Design review of the part shown in the three views and the two pictorial views. Dimensions are in mm from the part's minimum x, y and z. Coordinates: 2 decimals unless noted, no trailing zeros. Order: outer loops, then holes, each group sorted by start corner. A loop starts at its lowest first (then second) coordinate and runs counter-clockwise, first axis right, second up. Notation, with made-up numbers: (11.5, -2.75) -> (60.5, -2.75) arc R34 cw to (60.5, 29.25) -> close; hole circle Ø5 at (68.25, 42). An arc over 180 degrees is marked (long way). Write item = value, one per line. Start each with the question number.
1) Consider section C-C on z = 7. Give the boundary of the cut face in (x, y), and give its area (3 significant figures).
2) Insertion check: pin 1 Ø2 at (y, z) = (63, 6) entering from -X; pin 2 Ø2 at (x, z) = (31.5, 7) entering from -Y; pin 3 Ø4 at (x, z) = (16.5, 4.5) entering from +Y. Each pin has a flat end and moves straight along its axis. Give the tip position at first contact, or say it passes through.
3) Draft analysis for pull direction X (two halves, no side actions). For the marked faces 1, 2 and 3, state which applies: +X half, -X half, draft (parallel to the pull), parting line (faces both ways), or undercut.
4) Consider section A-A on y = 35. Give the boundary of the cut face in (x, z).
5) Wall thickness on probe 1 along Y at (x, z) = (35, 4.75); probe 2 along X at (y, z) = (30.5, 9) (1 decimal); probe 3 along X at (y, z) = (15, 9) (1 decimal): over which ranges is each line inside the solid? List them lowest first. Write a range as [from, to].
6) Consider section D-D on x = 48. Give the boundary of the cut face in (y, z), and give its area (3 significant figures).
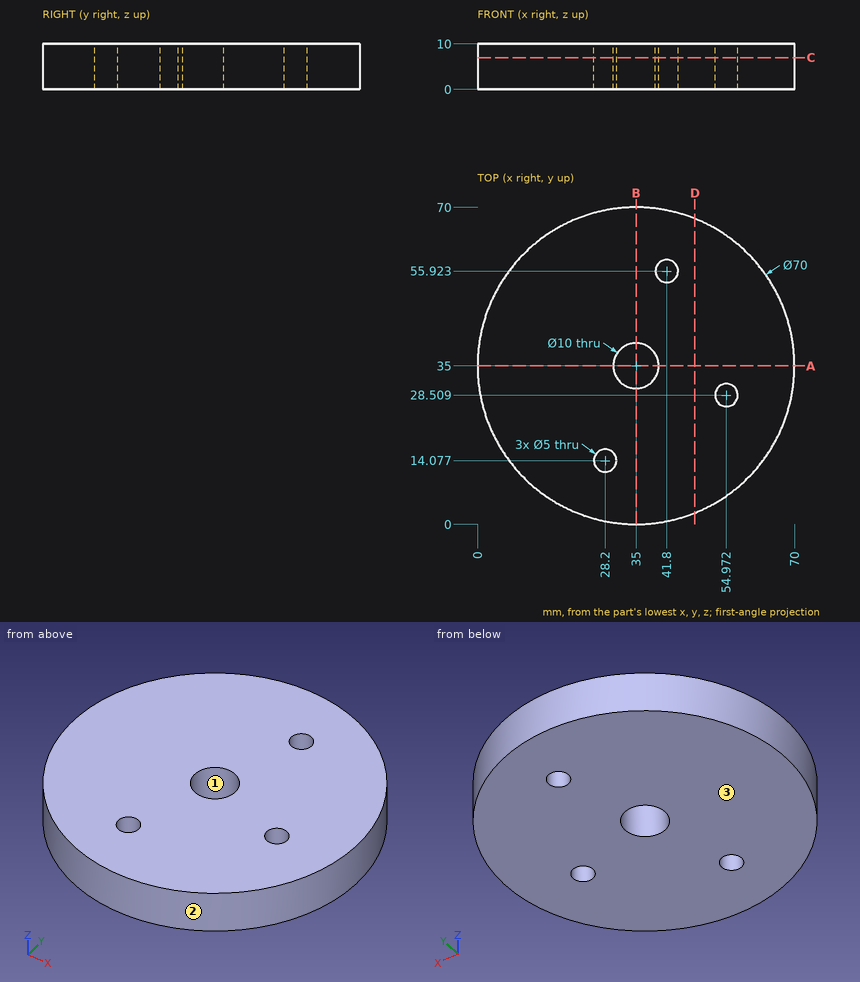
Answer sheet:
q1.outline = circle Ø70 at (35, 35); hole circle Ø5 at (28.2, 14.08); hole circle Ø10 at (35, 35); hole circle Ø5 at (41.8, 55.92); hole circle Ø5 at (54.97, 28.51)
q1.area = 3,710 mm2
q2.pin_1 = 12.73
q2.pin_2 = 0.09
q2.pin_3 = 65.87
q3.face_1 = undercut
q3.face_2 = parting line
q3.face_3 = draft
q4.outline = (0, 0) -> (30, 0) -> (30, 10) -> (0, 10) -> close; (40, 0) -> (70, 0) -> (70, 10) -> (40, 10) -> close
q5.probe_1 = [0, 30], [40, 70]
q5.probe_2 = [0.3, 32.8], [37.2, 53.5], [56.5, 69.7]
q5.probe_3 = [6.3, 25.9], [30.5, 63.7]
q6.outline = (2.5, 0) -> (67.5, 0) -> (67.5, 10) -> (2.5, 10) -> close
q6.area = 650 mm2
